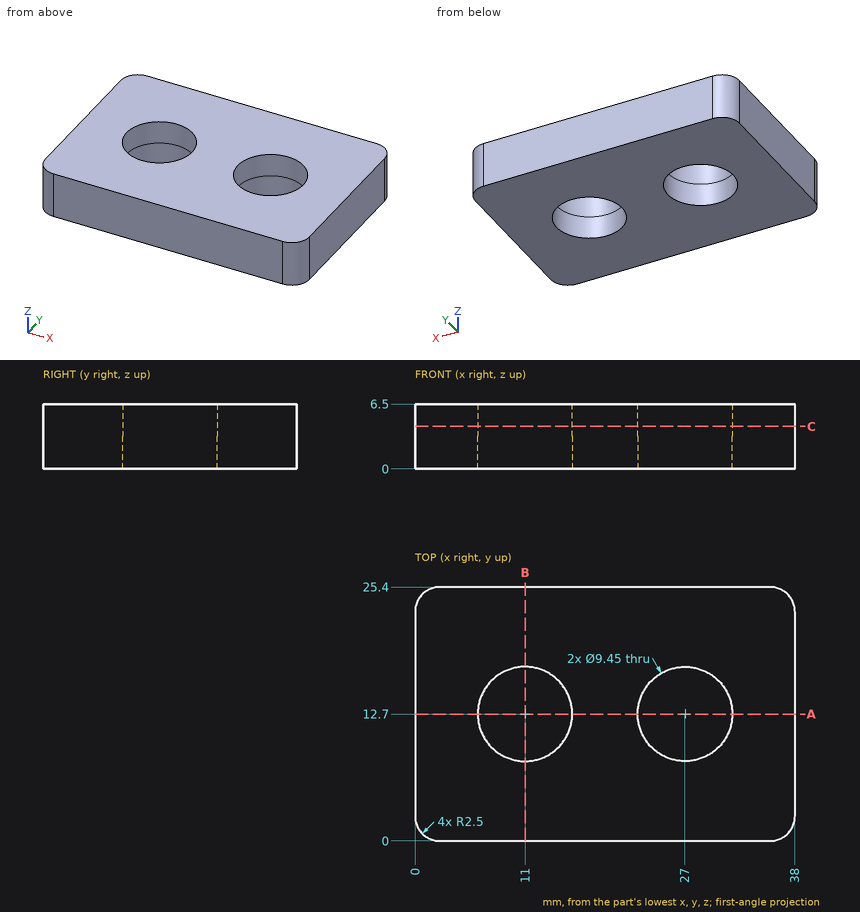
Answer from the drawing. Dimensions are ordinates in mm from the lowest x, y and z of the part. Coordinates: 2 decimals unless noted, no trailing zeros. Loops run counter-clockwise (first coordinate to the right, second up) from the corner with the lowest first, then second, coordinate; pieces in that order, holes last.
1) Section A-A (y = 12.7) is taken. Give the vertices of the cut face in (x, z) (3 decimals), plus the area to 3 significant figures.
Results:
outline: (0, 0) - (6.275, 0) - (6.275, 6.5) - (0, 6.5) - close; (15.725, 0) - (22.275, 0) - (22.275, 6.5) - (15.725, 6.5) - close; (31.725, 0) - (38, 0) - (38, 6.5) - (31.725, 6.5) - close
area: 124 mm2
2) Section B-B (x = 11) is taken. Give the vertices of the cut face in (y, z) (3 decimals), plus the area to 3 significant figures.
Results:
outline: (0, 0) - (7.975, 0) - (7.975, 6.5) - (0, 6.5) - close; (17.425, 0) - (25.4, 0) - (25.4, 6.5) - (17.425, 6.5) - close
area: 104 mm2
3) Consider probe 1 along Y at (x, z) = (27, 1.35) (3 decimals); probe 2 along X at (y, z) = (10.75, 2.25); probe 3 along X at (y, z) = (8.5, 4.75). Determine where each line is inside the solid, lowest interval first.
Results:
probe 1: y = 0 to 7.975, 17.425 to 25.4
probe 2: x = 0 to 6.7, 15.3 to 22.7, 31.3 to 38
probe 3: x = 0 to 8.84, 13.16 to 24.84, 29.16 to 38
4) A flat-ended cylindrical pin translates along its axis: pin 1 (12.5 mm diameter, centred on x = 11, y = 12.7, fed in from -Z). Find the tip coordinate at first contact, or state that the pin passes through.
Results:
pin 1: stops at z = 0
5) Section C-C (z = 4.25) is taken. Give the vertices of the cut face in (x, y) (3 decimals).
Results:
outline: (0, 2.5) arc R2.5 ccw to (2.5, 0) - (35.5, 0) arc R2.5 ccw to (38, 2.5) - (38, 22.9) arc R2.5 ccw to (35.5, 25.4) - (2.5, 25.4) arc R2.5 ccw to (0, 22.9) - close; hole circle Ø9.45 at (11, 12.7); hole circle Ø9.45 at (27, 12.7)
